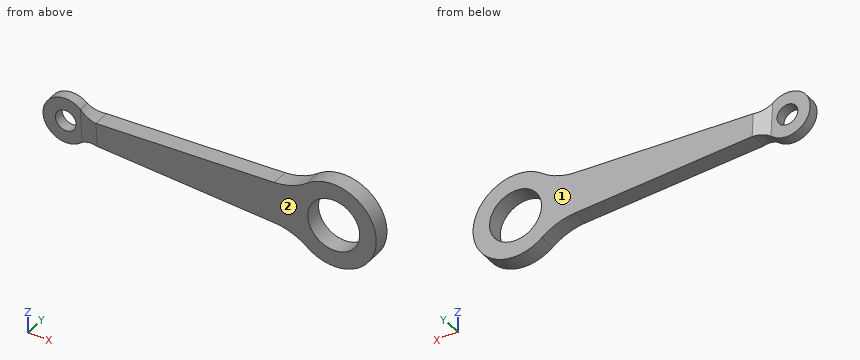
```python
from build123d import *

# Parameters (mm, degrees)
BOSS_EXTRUDE1_DEPTH      = 1.27
BOSS_EXTRUDE1_DEPTH_BACK = 1.27
SKETCH1_R                = 1.5875
SKETCH1_R_2              = 3.96875
CUT_EXTRUDE1_DEPTH       = 49.548015703
CUT_EXTRUDE1_DEPTH_BACK  = 49.548015703
CUT_EXTRUDE2_DEPTH       = 49.548015703
CUT_EXTRUDE2_DEPTH_BACK  = 49.548015703


with BuildPart() as part:
    # Sketch1 → Boss-Extrude1 (new, two sides: drawn at the far end of the back side and taken through both)
    with BuildSketch(Plane(origin=(0, 0, 0), x_dir=(1, 0, 0), z_dir=(0, 1, 0)).offset(-BOSS_EXTRUDE1_DEPTH_BACK)):
        with BuildLine():
            Line((4.906744273, 1.778), (32.198389451, 3.208294517))
            ThreePointArc((32.198389451, 3.208294517), (34.867586322, 3.767022283), (37.24183541, 5.108562416))
            ThreePointArc((37.24183541, 5.108562416), (47.78375, 0), (37.24183541, -5.108562416))
            ThreePointArc((37.24183541, -5.108562416), (34.867586322, -3.767022283), (32.198389451, -3.208294517))
            Line((32.198389451, -3.208294517), (4.906744273, -1.778))
            ThreePointArc((4.906744273, -1.778), (3.494086568, -1.971116067), (2.251338568, -2.670024513))
            ThreePointArc((2.251338568, -2.670024513), (-3.4925, 0), (2.251338568, 2.670024513))
            ThreePointArc((2.251338568, 2.670024513), (3.494086568, 1.971116067), (4.906744273, 1.778))
        make_face()
        with Locations(Location((0, 0, 0), (0, 0, 270))):
            Circle(SKETCH1_R, mode=Mode.SUBTRACT)
        with Locations(Location((41.275, 0, 0), (0, 0, 270))):
            Circle(SKETCH1_R_2, mode=Mode.SUBTRACT)
    extrude(amount=BOSS_EXTRUDE1_DEPTH + BOSS_EXTRUDE1_DEPTH_BACK)

    # Sketch2 → Cut-Extrude1 (cut, two sides: drawn at the far end of the back side and taken through both)
    with BuildSketch(Plane(origin=(-0.079485975, 0, 1.516682746), x_dir=(0.9986295347545739, 0, 0.05233595624294426), z_dir=(-0.05233595624294425, 0, 0.9986295347545738)).offset(-CUT_EXTRUDE1_DEPTH_BACK)):
        Polygon((-3.4925, 0.8001), (2.387991473, 0.8001), (4.99307308, 1.27), (4.99307308, 1.856442967), (-4.865374357, 1.856442967), align=None)
    extrude(amount=CUT_EXTRUDE1_DEPTH + CUT_EXTRUDE1_DEPTH_BACK, mode=Mode.SUBTRACT)

    # Sketch3 → Cut-Extrude2 (cut, two sides: drawn at the far end of the back side and taken through both)
    with BuildSketch(Plane(origin=(-0.079485975, 0, 1.516682746), x_dir=(0.9986295347545739, 0, 0.05233595624294426), z_dir=(-0.05233595624294425, 0, 0.9986295347545738)).offset(-CUT_EXTRUDE2_DEPTH_BACK)):
        Polygon((4.99307308, -1.27), (2.3495, -0.80386674), (-3.4925, -0.80386674), (-4.094294219, -2.202797579), (4.99307308, -2.202797579), align=None)
    extrude(amount=CUT_EXTRUDE2_DEPTH + CUT_EXTRUDE2_DEPTH_BACK, mode=Mode.SUBTRACT)


solid = part.part
```
Input: part model. Units: mm. Frame: model coordinates. Face numbers are marked on the shaded views. Round coordinates to 2 decimals unless told otherwise and drop trailing zeros. Loops run counter-clockwise (first coordinate to the right, second up) from the corner with the lowest first, then second, coordinate; pieces in that order, holes last. Notation, with made-up numbers: (-5, -35) -> (18, -35) arc R22 cw to (18, -26) -> close; hole circle Ø11 at (-15, -4). An arc over 180 degrees is marked (long way). Write each question's results on one line, items separated by ' | '.
1. First-contact query: P1, Ø5, axis at x = 0, z = 0, coming from the -Y side; P2, Ø6.5, axis at x = -0.5, z = 1, coming from the +Y side. Flat tips, straight axial feed; report the tip coordinate or a pass-through.
Geometry results:
P1: y = -0.83 | P2: y = 0.87
2. Mould query, pull axis Y, two halves, no side actions, for the marked faces 1 and 2. Classes: +Y half, -Y half, draft (parallel to the pull), parting line (faces both ways), or undercut.
Geometry results:
face 1: +Y half | face 2: -Y half
3. Section C-C (y = -0.05). Return loops of the section in (x, z) (1 decimal).
Geometry results:
outline: (2.3, -2.7) arc R3.8 cw to (4.9, -1.8) -> (32.2, -3.2) arc R8.9 cw to (37.2, -5.1) arc R6.5 ccw (long way) to (37.2, 5.1) arc R8.9 cw to (32.2, 3.2) -> (4.9, 1.8) arc R3.8 cw to (2.3, 2.7) arc R3.5 ccw (long way) to start; hole circle Ø3.2 at (0, 0); hole circle Ø7.9 at (41.3, 0)
4. Section A-A (x = 0). Return loops of the section in (y, z).
Geometry results:
outline: (-0.8, -3.49) -> (0.8, -3.49) -> (0.8, -1.59) -> (-0.8, -1.59) -> close; (-0.8, 1.59) -> (0.8, 1.59) -> (0.8, 3.49) -> (-0.8, 3.49) -> close
5. Section D-D (x = 17). Return loops of the section in (y, z), and give its area (3 significant figures).
Geometry results:
outline: (-1.27, -2.41) -> (1.27, -2.41) -> (1.27, 2.41) -> (-1.27, 2.41) -> close | area: 12.3 mm2
6. Section B-B (z = 0). Return loops of the section in (x, y).
Geometry results:
outline: (-3.49, -0.8) -> (-1.59, -0.8) -> (-1.59, 0.8) -> (-3.49, 0.8) -> close; (1.59, -0.8) -> (2.35, -0.8) -> (5, -1.27) -> (37.31, -1.27) -> (37.31, 1.27) -> (5, 1.27) -> (2.39, 0.8) -> (1.59, 0.8) -> close; (45.24, -1.27) -> (47.78, -1.27) -> (47.78, 1.27) -> (45.24, 1.27) -> close
7. Ray query, line 1 (Z direction, x = 0, y = -0.35); line 2 (X direction, y = -0.35, z = 0); line 3 (Z direction, x = 41.5, y = 1.05). Return the intervals inside material, ascending. Write a range as from..to.
Geometry results:
line 1: -3.49..-1.59, 1.59..3.49 | line 2: -3.49..-1.59, 1.59..37.31, 45.24..47.78 | line 3: -6.5..-3.96, 3.96..6.5
